Part model, mm, in its own coordinate system. A direction names the side the tool comes from. Coordinates: 2 decimals unless noted, no trailing zeros. Write each loop counter-clockwise with the first axis right and the second up, starting at its lowest first coordinate (ties: lowest second). Pieces come first, ordered by that corner, then holes. Notation, with made-up numbers: M 44.25,27 L 103.25,27 A21 ccw 103.25,37 Z; hole C -38,-20 d8. An arc over 180 degrees is marked long. Use a Markdown table: item, result. Add a question column.
Q1. Slice it at A-A on z = 7. Write the cut outline in (x, y).
Q2. Pin check, flat tip, straight feed: pin 1 Ø19.5 at (y, z) = (30.5, 18.5) entering from -X. Stop position of the tip, or through.
Q3. Slice it at C-C on x = -38. Write the cut outline in (y, z).
Q4. Slice it at B-B on y = 33. Write the cut outline in (x, z), then the cut area to 3 significant figures.
Q5. Tool access for faces 1 (the flat face through (-20.988, 11, 19)), 2 (the flat face through (7, 3, 38.849)): list every direction of +Z, -Z, +X, -X, +Y, -Y with a clear straight run to the whole face (end or side of a thin tool).
Q6. Wall check: L1, parallel to X at y = -25, z = 30; L2, parallel to Y at x = -34.5, z = 37. Give the ranges that are in metal, low to high. Write a range as from..to.
from build123d import *

# Parameters (mm, degrees)
F0_W      = 60.731009
F0_H      = 107.71951
F0_W_2    = 22.791378
F0_H_2    = 20.984024
F1_DEPTH  = 38.848586
F1_FACE_W = 20.984024
F1_FACE_H = 38.848586
F2_DEPTH  = 27.409891
F3_W      = 20.984024
F3_H      = 38.848586
F4_DEPTH  = 31.743571


with BuildPart() as f1:
    # F0 (on Top) → F1 (new body)
    with BuildSketch(Plane.XY):
        with Locations((9.377531, 12.187466)):
            Rectangle(F0_W, F0_H)
        with Locations((-32.383662, -52.164301)):
            Rectangle(F0_W_2, F0_H_2)
        with Locations((9.377531, -52.164301)):
            Rectangle(F0_W, F0_H_2)
    extrude(amount=F1_DEPTH)

    # F1_face (on face) → F2 (join)
    with BuildSketch(Plane(origin=(-43.779351, -52.164301, 19.424293), x_dir=(0, -1, 0), z_dir=(-1, 0, 0))):
        Rectangle(F1_FACE_W, F1_FACE_H)
    extrude(amount=-F2_DEPTH)

    # F3 (on face) → F4 (join)
    with BuildSketch(Plane(origin=(-43.779351, 0, 0), x_dir=(0, -1, 0), z_dir=(-1, 0, 0))):
        with Locations((52.164301, 19.424293)):
            Rectangle(F3_W, F3_H)
    extrude(amount=-F4_DEPTH)


solid = f1.part
Recorded:
| question | item | result |
|---|---|---|
| 1 | outline | M -43.78,-62.66 L 39.74,-62.66 L 39.74,66.05 L -20.99,66.05 L -20.99,-41.67 L -43.78,-41.67 Z |
| 2 | pin 1 | x = -20.99 |
| 3 | outline | M -62.66,0 L -41.67,0 L -41.67,38.85 L -62.66,38.85 Z |
| 4 | outline | M -20.99,0 L 39.74,0 L 39.74,38.85 L -20.99,38.85 Z |
| 4 | area | 2,360 mm² |
| 5 | face 1 | +Z, -Z, -X, +Y |
| 5 | face 2 | +Z, +X, -X, +Y, -Y |
| 6 | L1 | -20.99..39.74 |
| 6 | L2 | -62.66..-41.67 |
